from build123d import *

# Parameters (mm, degrees)
ESBO_O7_W                = 170
ESBO_O7_H                = 120
RESSALTO_EXTRUS_O4_DEPTH = 80
CORTE_EXTRUS_O9_DEPTH    = 30
CASCA1_T                 = -5
ESBO_O9_R                = 1.25
CORTE_EXTRUS_O4_DEPTH    = 132.244047484
CORTE_EXTRUS_O5_DEPTH    = 2.5
ESBO_O13_R               = 4
CORTE_EXTRUS_O7_DEPTH    = 132.244047484
CORTE_EXTRUS_O8_DEPTH    = 2.5
ESBO_O22_W               = 14
ESBO_O22_H               = 20.5
CORTE_EXTRUS_O10_DEPTH   = 193.937813816
ESBO_O23_W               = 10
ESBO_O23_H               = 50
CORTE_EXTRUS_O11_DEPTH   = 193.937813816
CHANFRO1_SIZE            = 2
FILETE2_R                = 3
ESBO_O25_W               = 164.4
ESBO_O25_H               = 114.4
CORTE_EXTRUS_O12_DEPTH   = 5
ESBO_O26_R               = 1
CORTE_EXTRUS_O13_DEPTH   = 168.406690428
ESBO_O27_W               = 10
ESBO_O27_H               = 10
ESBO_O27_R               = 1
RESSALTO_EXTRUS_O7_DEPTH = 10
CHANFRO2_SIZE            = 2


with BuildPart() as part:
    # Esbo_o7 → Ressalto-extrus_o4 (new body)
    with BuildSketch(Plane(origin=(0, 0, 0), x_dir=(1, 0, 0), z_dir=(0, 1, 0))):
        Rectangle(ESBO_O7_W, ESBO_O7_H)
    extrude(amount=RESSALTO_EXTRUS_O4_DEPTH)

    # Esbo_o17 → Corte-extrus_o9 (cut)
    with BuildSketch(Plane.XY.offset(60)):
        Polygon((-85, 25.75), (-33.281920983, 25.75), (-18.415151551, 0), (-85, 0), align=None)
        Polygon((85, 0), (18.415151551, 0), (33.281920983, 25.75), (85, 25.75), align=None)
    corte_extrus_o9 = extrude(amount=-CORTE_EXTRUS_O9_DEPTH, mode=Mode.SUBTRACT)

    # Espelhar3: Corte-extrus_o9 across plane
    add(corte_extrus_o9.mirror(Plane.XY), mode=Mode.SUBTRACT)

    # Casca1
    casca1_openings = [part.faces().sort_by_distance(p)[0] for p in [
        (0, 80, 0),
    ]]
    offset(amount=CASCA1_T, openings=casca1_openings, kind=Kind.INTERSECTION)

    # Esbo_o9 → Corte-extrus_o4 (cut, through all)
    with BuildSketch(Plane.XZ):
        with Locations(Location((40.35, -13.25, 0), (0, 0, 270))):
            Circle(ESBO_O9_R)
        with Locations(Location((32.65, -13.25, 0), (0, 0, 270))):
            Circle(ESBO_O9_R)
        with Locations(Location((40.35, 13.25, 0), (0, 0, 270))):
            Circle(ESBO_O9_R)
        with Locations(Location((32.65, 13.25, 0), (0, 0, 270))):
            Circle(ESBO_O9_R)
        with Locations(Location((-30.15, 13.25, 0), (0, 0, 270))):
            Circle(ESBO_O9_R)
        with Locations(Location((-37.85, 13.25, 0), (0, 0, 270))):
            Circle(ESBO_O9_R)
        with Locations(Location((-30.15, -13.25, 0), (0, 0, 270))):
            Circle(ESBO_O9_R)
        with Locations(Location((-37.85, -13.25, 0), (0, 0, 270))):
            Circle(ESBO_O9_R)
    extrude(amount=-CORTE_EXTRUS_O4_DEPTH, mode=Mode.SUBTRACT)

    # Esbo_o10 → Corte-extrus_o5 (cut)
    with BuildSketch(Plane(origin=(0, 5, 0), x_dir=(1, 0, 0), z_dir=(0, 1, 0))):
        with BuildLine():
            Line((41.35, 16.25), (31.65, 16.25))
            ThreePointArc((31.65, 16.25), (30.235786438, 15.664213562), (29.65, 14.25))
            Line((29.65, 14.25), (29.65, -14.25))
            ThreePointArc((29.65, -14.25), (30.235786438, -15.664213562), (31.65, -16.25))
            Line((31.65, -16.25), (41.35, -16.25))
            ThreePointArc((41.35, -16.25), (42.764213562, -15.664213562), (43.35, -14.25))
            Line((43.35, -14.25), (43.35, 14.25))
            ThreePointArc((43.35, 14.25), (42.764213562, 15.664213562), (41.35, 16.25))
        make_face()
        with BuildLine():
            Line((-38.85, 16.25), (-29.15, 16.25))
            ThreePointArc((-29.15, 16.25), (-27.735786438, 15.664213562), (-27.15, 14.25))
            Line((-27.15, 14.25), (-27.15, -14.25))
            ThreePointArc((-27.15, -14.25), (-27.735786438, -15.664213562), (-29.15, -16.25))
            Line((-29.15, -16.25), (-38.85, -16.25))
            ThreePointArc((-38.85, -16.25), (-40.264213562, -15.664213562), (-40.85, -14.25))
            Line((-40.85, -14.25), (-40.85, 14.25))
            ThreePointArc((-40.85, 14.25), (-40.264213562, 15.664213562), (-38.85, 16.25))
        make_face()
    extrude(amount=-CORTE_EXTRUS_O5_DEPTH, mode=Mode.SUBTRACT)

    # Esbo_o13 → Corte-extrus_o7 (cut, through all)
    with BuildSketch(Plane(origin=(0, 80, 0), x_dir=(1, 0, 0), z_dir=(0, 1, 0))):
        with Locations(Location((0, 0, 0), (0, 0, 270))):
            Circle(ESBO_O13_R)
    extrude(amount=-CORTE_EXTRUS_O7_DEPTH, mode=Mode.SUBTRACT)

    # Esbo_o14 → Corte-extrus_o8 (cut)
    with BuildSketch(Plane(origin=(0, 5, 0), x_dir=(1, 0, 0), z_dir=(0, 1, 0))):
        with BuildLine():
            Line((-4.5, -30), (-4.5, 30))
            ThreePointArc((-4.5, 30), (0, 34.5), (4.5, 30))
            Line((4.5, 30), (4.5, -30))
            ThreePointArc((4.5, -30), (0, -34.5), (-4.5, -30))
        make_face()
    extrude(amount=-CORTE_EXTRUS_O8_DEPTH, mode=Mode.SUBTRACT)

    # Esbo_o22 → Corte-extrus_o10 (cut, through all)
    with BuildSketch(Plane.ZY.offset(-80)):
        Polygon((43.24, 57.45), (32.12, 57.45), (31.66, 57.45), (31.66, 56.89), (31.66, 47.24), (32.12, 47.24), (43.24, 47.24), (43.7, 47.24), (43.7, 56.89), (43.7, 57.45), align=None)
        with Locations((-26.5, 57)):
            Rectangle(ESBO_O22_W, ESBO_O22_H)
    extrude(amount=-CORTE_EXTRUS_O10_DEPTH, mode=Mode.SUBTRACT)

    # Esbo_o23 → Corte-extrus_o11 (cut, through all)
    with BuildSketch(Plane(origin=(-80, 0, 0), x_dir=(0, 0, -1), z_dir=(1, 0, 0))):
        with Locations((-15, 55)):
            Rectangle(ESBO_O23_W, ESBO_O23_H)
        with Locations((15, 55)):
            Rectangle(ESBO_O23_W, ESBO_O23_H)
    extrude(amount=-CORTE_EXTRUS_O11_DEPTH, mode=Mode.SUBTRACT)

    # Chanfro1
    chanfro1_edges = [part.edges().sort_by_distance(p)[0] for p in [
        (-80, 55, 10),
        (-80, 55, 20),
        (-80, 55, -10),
        (-80, 55, -20),
    ]]
    chamfer(chanfro1_edges, length=CHANFRO1_SIZE)

    # Filete2
    filete2_edges = [part.edges().sort_by_distance(p)[0] for p in [
        (-85, 12.875, 30),
        (-25.848536267, 12.875, 30),
        (-25.848536267, 12.875, 60),
        (85, 12.875, 30),
        (25.848536267, 12.875, 30),
        (25.848536267, 12.875, 60),
        (-25.848536267, 12.875, -60),
        (-85, 12.875, -30),
        (-25.848536267, 12.875, -30),
        (25.848536267, 12.875, -60),
        (85, 12.875, -30),
        (25.848536267, 12.875, -30),
        (-85, 52.875, -60),
        (85, 52.875, -60),
        (85, 52.875, 60),
        (-85, 52.875, 60),
    ]]
    fillet(filete2_edges, radius=FILETE2_R)

    # Esbo_o25 → Corte-extrus_o12 (cut)
    with BuildSketch(Plane(origin=(0, 80, 0), x_dir=(1, 0, 0), z_dir=(0, 1, 0))):
        Rectangle(ESBO_O25_W, ESBO_O25_H)
    extrude(amount=-CORTE_EXTRUS_O12_DEPTH, mode=Mode.SUBTRACT)

    # Esbo_o26 → Corte-extrus_o13 (cut, through all)
    with BuildSketch(Plane(origin=(0, 0, -60), x_dir=(-1, 0, 0), z_dir=(0, 0, -1))):
        with Locations((-79.35, 77.5)):
            Circle(ESBO_O26_R)
        with Locations((79.35, 77.5)):
            Circle(ESBO_O26_R)
    extrude(amount=-CORTE_EXTRUS_O13_DEPTH, mode=Mode.SUBTRACT)

    # Esbo_o27 → Ressalto-extrus_o7 (add)
    # profile 1 of 4: a face of its own
    with BuildSketch(Plane(origin=(0, 30.75, 0), x_dir=(1, 0, 0), z_dir=(0, 1, 0))):
        with Locations((-75, 50)):
            Rectangle(ESBO_O27_W, ESBO_O27_H)
        with Locations(Location((-75, 50, 0), (0, 0, 180))):
            Circle(ESBO_O27_R, mode=Mode.SUBTRACT)
    # profile 2 of 4: a face of its own
    with BuildSketch(Plane(origin=(0, 30.75, 0), x_dir=(1, 0, 0), z_dir=(0, 1, 0))):
        with Locations((75, 50)):
            Rectangle(ESBO_O27_W, ESBO_O27_H)
        with Locations(Location((75, 50, 0), (0, 0, 180))):
            Circle(ESBO_O27_R, mode=Mode.SUBTRACT)
    # profile 3 of 4: a face of its own
    with BuildSketch(Plane(origin=(0, 30.75, 0), x_dir=(1, 0, 0), z_dir=(0, 1, 0))):
        with Locations((75, -50)):
            Rectangle(ESBO_O27_W, ESBO_O27_H)
        with Locations(Location((75, -50, 0), (0, 0, 180))):
            Circle(ESBO_O27_R, mode=Mode.SUBTRACT)
    # profile 4 of 4: a face of its own
    with BuildSketch(Plane(origin=(0, 30.75, 0), x_dir=(1, 0, 0), z_dir=(0, 1, 0))):
        with Locations((-75, -50)):
            Rectangle(ESBO_O27_W, ESBO_O27_H)
        with Locations(Location((-75, -50, 0), (0, 0, 180))):
            Circle(ESBO_O27_R, mode=Mode.SUBTRACT)
    extrude(amount=RESSALTO_EXTRUS_O7_DEPTH)

    # Chanfro2
    chanfro2_edges = [part.edges().sort_by_distance(p)[0] for p in [
        (85, 57.45, 37.68),
        (85, 52.345, 31.66),
        (85, 52.345, 43.7),
        (85, 47.24, 37.68),
        (85, 57, -19.5),
        (85, 46.75, -26.5),
        (85, 57, -33.5),
        (85, 67.25, -26.5),
    ]]
    chamfer(chanfro2_edges, length=CHANFRO2_SIZE)


solid = part.part
The model under review builds one solid part; all positions refer to its coordinate system, in mm. A direction names the side the tool comes from. Give positions to 0.01 mm unless a question says otherwise; leave off trailing zeros. Write each loop counter-clockwise with the first axis right and the second up, starting at its lowest first coordinate (ties: lowest second). Pieces come first, ordered by that corner, then holes.
1. For P1, Ø2, axis at x = -34, y = 4.5, coming from the +Z side; P2, Ø3, axis at x = -36, z = -30.5, coming from the +Y side; P3, Ø7.5, axis at x = 49.5, y = 15, coming from the -Z side, all flat-tipped, find the tip position at first contact; note any pin that passes through.
2. Add section B-B, the plane x = 60. Write out the cut boundary in (y, z), plus the area to 3 significant figures.
3. Add section A-A, the plane z = 0. Write out the cut boundary in (x, y), plus the area to 3 significant figures.
4. Wall thickness on L1, parallel to X at y = 1, z = 13; L2, parallel to Z at x = 75, y = 38; L3, parallel to Z at x = 15, y = 8.5: over which ranges is each line inside the solid? List them lowest first.
5. Draft analysis for pull direction Z (two halves, no side actions). For faces 1 (the flat face through (-85, 39, 1)), 2 (the cylindrical face through (24.78, 12.74, 59.1)), 3 (the flat face through (80, 47, 1)), state which applies: +Z half, -Z half, draft (parallel to the pull), parting line (faces both ways), or undercut.
6. Tool access review of faces 4 (the flat face through (-1, 78, -57.2)), 5 (the flat face through (-58, 25.75, -47)): name each direction out of +Z, -Z, +X, -X, +Y, -Y from which nothing blocks a thin tool from reaching the whole face with its end or side.
Worked answers:
1. P1: stops at z = 30
1. P2: stops at y = 30.75
1. P3: stops at z = -30
2. outline: (0, -30) - (25.75, -30) - (25.75, -60) - (80, -60) - (80, -57.2) - (75, -57.2) - (75, -55) - (30.75, -55) - (30.75, -25) - (5, -25) - (5, 25) - (30.75, 25) - (30.75, 55) - (75, 55) - (75, 57.2) - (80, 57.2) - (80, 60) - (25.75, 60) - (25.75, 30) - (0, 30) - close
2. area: 1,330 mm2
3. outline: (-85, 0) - (-4, 0) - (-4, 2.5) - (-4.5, 2.5) - (-4.5, 5) - (-27.15, 5) - (-27.15, 2.5) - (-40.85, 2.5) - (-40.85, 5) - (-80, 5) - (-80, 75) - (-82.2, 75) - (-82.2, 80) - (-85, 80) - close; (4, 0) - (85, 0) - (85, 80) - (82.2, 80) - (82.2, 75) - (80, 75) - (80, 5) - (43.35, 5) - (43.35, 2.5) - (29.65, 2.5) - (29.65, 5) - (4.5, 5) - (4.5, 2.5) - (4, 2.5) - close
3. area: 1,470 mm2
4. L1: x = -85 to -39.07, -36.63 to -31.37, -28.93 to 31.43, 33.87 to 39.13, 41.57 to 85
4. L2: z = -60 to -51, -49 to -45, 45 to 49, 51 to 60
4. L3: z = -60 to -55, 55 to 60
5. face 1: draft
5. face 2: +Z half
5. face 3: undercut
6. face 4: +Y
6. face 5: -Z, -X, -Y
